Work out the finished part from the listing and answer in its coordinate system (mm). Face numbers are marked on the shaded views. A direction names the side the tool comes from. Give positions to 0.01 mm unless a question says otherwise; leave off trailing zeros. Order: outer loops, then holes, each group sorted by start corner. A loop starts at its lowest first (then second) coordinate and runs counter-clockwise, first axis right, second up. Notation, with made-up numbers: M 23,-14.5 L 79,-14.5 A20 ccw 79,14.5 Z; hole C 76,-35.75 d6. An arc over 180 degrees is marked long. One line per item, written item: value.
from build123d import *

# Parameters (mm, degrees)
RESSALTO_EXTRUS_O1_DEPTH   = 40
ESBO_O2_R                  = 1.65
ESBO_O2_R_2                = 9
CORTE_EXTRUS_O1_DEPTH      = 19
CORTE_EXTRUS_O1_DEPTH_BACK = 9
ESBO_O3_R                  = 1.65
CORTE_EXTRUS_O2_DEPTH      = 39.3
ESBO_O4_R                  = 11.05
CORTE_EXTRUS_O3_DEPTH      = 7
CORTE_EXTRUS_O5_START      = 7
ESBO_O7_R                  = 5.25
CORTE_EXTRUS_O5_DEPTH      = 10
FILETE1_R                  = 8
ESBO_O8_R                  = 5.25
CORTE_EXTRUS_O6_DEPTH      = 1
ESBO_O7_2_R                = 5.25
CORTE_EXTRUS_O7_DEPTH      = 1


with BuildPart() as part:
    # Esboço1 → Ressalto-extrusão1 (new body)
    with BuildSketch(Plane.XY):
        Polygon((0, 0), (6, 0), (12.551464217, 18), (49, 18), (49, 26), (-20, 26), (-20, 20), (0, 20), align=None)
    extrude(amount=RESSALTO_EXTRUS_O1_DEPTH)

    # Esboço2 → Corte-extrusão1 (cut, two sides)
    with BuildSketch(Plane.XZ.offset(-18)) as corte_extrus_o1_sk:
        with Locations((-10, 11)):
            Circle(ESBO_O2_R)
        with Locations((21.3, 20)):
            Circle(ESBO_O2_R_2)
        with Locations((-10, 29)):
            Circle(ESBO_O2_R)
        with BuildLine():
            Line((21.3, 3), (-20, 3))
            Line((-20, 3), (-20, 0))
            Line((-20, 0), (49, 0))
            Line((49, 0), (49, 40))
            Line((49, 40), (-20, 40))
            Line((-20, 40), (-20, 37))
            Line((-20, 37), (21.3, 37))
            ThreePointArc((21.3, 37), (38.3, 20), (21.3, 3))
        make_face()
    extrude(amount=CORTE_EXTRUS_O1_DEPTH, mode=Mode.SUBTRACT)
    extrude(corte_extrus_o1_sk.sketch, amount=-CORTE_EXTRUS_O1_DEPTH_BACK, mode=Mode.SUBTRACT)

    # Esboço3 → Corte-extrusão2 (cut, through all)
    with BuildSketch(Plane.ZY):
        with Locations((29, 10)):
            Circle(ESBO_O3_R)
        with Locations((11, 10)):
            Circle(ESBO_O3_R)
    extrude(amount=-CORTE_EXTRUS_O2_DEPTH, mode=Mode.SUBTRACT)

    # Esboço4 → Corte-extrusão3 (cut)
    with BuildSketch(Plane(origin=(0, 26, 0), x_dir=(1, 0, 0), z_dir=(0, 1, 0))):
        with Locations((21.3, -20)):
            Circle(ESBO_O4_R)
    extrude(amount=-CORTE_EXTRUS_O3_DEPTH, mode=Mode.SUBTRACT)

    # Esboço7 → Corte-extrusão5 (cut)
    with BuildSketch(Plane(origin=(0, 0, 0), x_dir=(0, 0, -1), z_dir=(1, 0, 0)).offset(CORTE_EXTRUS_O5_START)):
        with Locations((-29, 10)):
            Circle(ESBO_O7_R)
        with Locations((-11, 10)):
            Circle(ESBO_O7_R)
    extrude(amount=CORTE_EXTRUS_O5_DEPTH, mode=Mode.SUBTRACT)

    # Filete1
    filete1_edges = [part.edges().sort_by_distance(p)[0] for p in [
        (-20, 23, 3),
        (-20, 23, 37),
        (3, 0, 37),
        (3, 0, 3),
    ]]
    fillet(filete1_edges, radius=FILETE1_R)

    # Esboço8 → Corte-extrusão6 (cut)
    with BuildSketch(Plane.XZ.offset(-20)):
        with Locations((-10, 11)):
            Circle(ESBO_O8_R)
        with Locations((-10, 29)):
            Circle(ESBO_O8_R)
    extrude(amount=-CORTE_EXTRUS_O6_DEPTH, mode=Mode.SUBTRACT)

    # Esboço7<2> → Corte-extrusão7 (cut)
    with BuildSketch(Plane(origin=(0, 0, 0), x_dir=(0, 0, -1), z_dir=(1, 0, 0))):
        with Locations((-29, 10)):
            Circle(ESBO_O7_2_R)
        with Locations((-11, 10)):
            Circle(ESBO_O7_2_R)
    extrude(amount=CORTE_EXTRUS_O7_DEPTH, mode=Mode.SUBTRACT)


solid = part.part
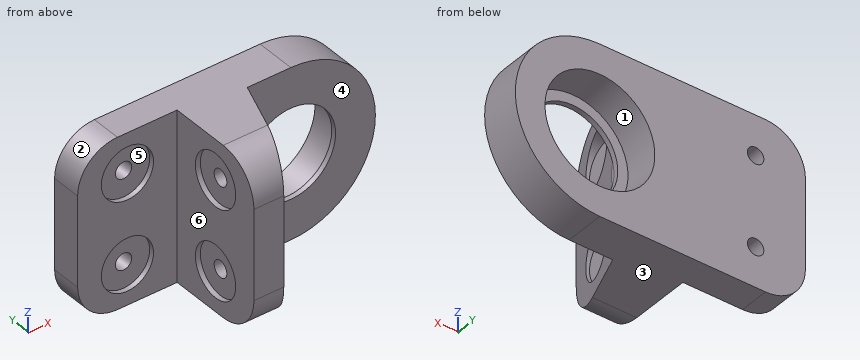
(1) Section A-A, the plane x = -10 is taken. Give the vertices of the cut face in (y, z), then the cut area to 3 significant figures.
Findings:
outline: M 20,3 L 26,3 L 26,9.35 L 21,9.35 L 21,5.75 L 20,5.75 Z; M 20,16.25 L 21,16.25 L 21,12.65 L 26,12.65 L 26,27.35 L 21,27.35 L 21,23.75 L 20,23.75 Z; M 20,34.25 L 21,34.25 L 21,30.65 L 26,30.65 L 26,37 L 20,37 Z
area: 150 mm^2
(2) Find the intervals of material crossed by probe 1 along X at (y, z) = (23, 29.5); probe 2 along Z at (x, y) = (-10, 24.55); probe 3 along Y at (x, z) = (3, 29), in increasing order. Write a range as from..to.
Findings:
probe 1: x = -19.98..-11.57, -8.43..15.66, 26.94..35.4
probe 2: z = 3..9.35, 12.65..27.35, 30.65..37
probe 3: y = 0..8.35, 11.65..26
(3) Section D-D, the plane z = 33 is taken. Give the vertices of the cut face in (x, y), then the cut area to 3 significant figures.
Findings:
outline: M -18.93,20 L -13.4,20 L -13.4,21 L -6.6,21 L -6.6,20 L 0,20 L 0,13.4 L 1,13.4 L 1,6.6 L 0,6.6 L 0,1.07 L 6.39,1.07 L 8.4,6.6 L 7,6.6 L 7,13.4 L 10.88,13.4 L 12.55,18 L 32.25,18 L 32.25,26 L -18.93,26 Z
area: 500 mm^2
(4) Which of the six approach directions +Z, -Z, +X, -X, +Y, -Y give full straight-line access (tool end or side, diameter ignored) to the marked faces 4, 5 and 6?
Findings:
face 4: +Z, -Z, +X, -Y
face 5: -Y
face 6: +Z, -Z, -X, -Y
(5) Section B-B, the plane z = 20 is taken. Give the vertices of the cut face in (x, y), then the cut area to 3 significant figures.
Findings:
outline: M -20,20 L 0,20 L 0,0 L 6,0 L 12.3,17.31 L 12.3,19 L 10.25,19 L 10.25,26 L -20,26 Z; M 30.3,18 L 38.3,18 L 38.3,26 L 32.35,26 L 32.35,19 L 30.3,19 Z
area: 421 mm^2
(6) Section C-C, the plane y = 10 is taken. Give the vertices of the cut face in (x, z).
Findings:
outline: M 0,3 L 9.64,3 L 9.64,5.75 L 7,5.75 L 7,9.35 L 1,9.35 L 1,5.75 L 0,5.75 Z; M 0,16.25 L 1,16.25 L 1,12.65 L 7,12.65 L 7,16.25 L 9.64,16.25 L 9.64,23.75 L 7,23.75 L 7,27.35 L 1,27.35 L 1,23.75 L 0,23.75 Z; M 0,34.25 L 1,34.25 L 1,30.65 L 7,30.65 L 7,34.25 L 9.64,34.25 L 9.64,37 L 0,37 Z
(7) Given P1, Ø3, axis at y = 9.5, z = 31, coming from the +X side; P2, Ø8.5, axis at y = 10, z = 11, coming from the -X side; P3, Ø8, axis at y = 11, z = 19, coming from the -X side, each flat-ended and moving along its own axis, determine where each tip first touches the part or whether it passes through.
Findings:
P1: stops at x = 7
P2: stops at x = 1
P3: stops at x = 0
(8) Determine the mould class of the marked faces 1, 2 and 3 for opening direction X: pulls with the +X half, pulls with the -X half, needs draft (parallel to the pull), parting line crosses it, or undercut.
Findings:
face 1: undercut
face 2: pulls with the -X half
face 3: needs draft
